Work out the finished part from the listing and answer in its coordinate system (mm). A direction names the side the tool comes from. Coordinates: 2 decimals unless noted, no trailing zeros. Order: outer loops, then holes, each group sorted by start corner. A loop starts at its lowest first (then second) coordinate and runs counter-clockwise, first axis right, second up.
```python
from build123d import *

# Parameters (mm, degrees)
SKETCH_1_W      = 5
SKETCH_1_H      = 5
SKETCH_1_W_2    = 3
SKETCH_1_H_2    = 3
EXTRUDE_1_DEPTH = 8
SKETCH_2_W      = 5
SKETCH_2_H      = 5
EXTRUDE_2_DEPTH = 2
SKETCH_3_W      = 10
SKETCH_3_H      = 2
EXTRUDE_3_DEPTH = 2
EXTRUDE_4_DEPTH = 2


with BuildPart() as part:
    # 草图1 → 凸台-拉伸1 (new body)
    with BuildSketch(Plane(origin=(0, 0, 0), x_dir=(0, 0, -1), z_dir=(1, 0, 0))):
        Rectangle(SKETCH_1_W, SKETCH_1_H)
        Rectangle(SKETCH_1_W_2, SKETCH_1_H_2, mode=Mode.SUBTRACT)
    extrude(amount=EXTRUDE_1_DEPTH)

    # 草图2 → 凸台-拉伸2 (add)
    with BuildSketch(Plane(origin=(8, 0, 0), x_dir=(0, 0, -1), z_dir=(1, 0, 0))):
        Rectangle(SKETCH_2_W, SKETCH_2_H)
    extrude(amount=EXTRUDE_2_DEPTH)

    # 草图3 → 凸台-拉伸3 (add)
    with BuildSketch(Plane.XZ.offset(2.5)):
        with Locations((5, 0)):
            Rectangle(SKETCH_3_W, SKETCH_3_H)
    extrude(amount=EXTRUDE_3_DEPTH)

    # 草图4 → 凸台-拉伸4 (add)
    with BuildSketch(Plane.XY.offset(1)):
        with BuildLine():
            Line((10, -4.5), (0, -4.5))
            Line((0, -4.5), (1.040402547, -12.634344629))
            ThreePointArc((1.040402547, -12.634344629), (8.203170669, -16.488433915), (9.535533906, -8.464466094))
            ThreePointArc((9.535533906, -8.464466094), (7.767766953, -8.464466094), (7.767766953, -10.232233047))
            ThreePointArc((7.767766953, -10.232233047), (5.996135796, -14.499997014), (4.237706296, -10.226776691))
            Line((4.237706296, -10.226776691), (7.30901916, -7.174394459))
            Line((7.30901916, -7.174394459), (10, -4.5))
        make_face()
    extrude(amount=-EXTRUDE_4_DEPTH)


solid = part.part
```
1. The part is cut by section C-C (y = 0.5). Determine the outline of the cut face in (x, z), plus the area to 3 significant figures.
2. For faces 4 (the flat face through (5, -8, -1)), 5 (the cylindrical face through (8.083, -16.545, 0.014)), 6 (the flat face through (5, 0, -2.5)), 7 (the flat face through (5, -2.5, 2)), 8 (the flat face through (4, 1.5, 0)), determine the directions among +Z, -Z, +X, -X, +Y, -Y from which every point of the face is accessible in a straight line to the end or side of a thin tool.
3. The part is cut by section A-A (x = 6). Determine the outline of the cut face in (y, z).
4. The part is cut by section D-D (z = 0.8). Determine the outline of the cut face in (x, y).
5. The part is cut by section B-B (y = -12). Determine the outline of the cut face in (x, z), plus the area to 3 significant figures.
6. Consider probe 1 along Z at (x, y) = (6, -0.75); probe 2 along Y at (x, z) = (6, 0.4); probe 3 along Y at (x, z) = (6.5, 0.3). Determine where each line is inside the solid, lowest interval first.
7. The mould has two halves that part along X. Classify faces 1 (the cylindrical face through (7.787, -8.445, 0.014)), 2 (the flat face through (5, 2.5, 0)), 3 (the flat face through (10, 0, 0)): released by +X, released by -X, zero draft, split by the parting line, or undercut.
8. Flat-ended cylindrical pins translate along their axes: pin 1 (5 mm diameter, centred on x = 7, y = -10, fed in from +Z); pin 2 (2 mm diameter, centred on y = -6, z = -0.5, fed in from -X); pin 3 (1.6 mm diameter, centred on x = 6.5, z = -2, fed in from -Y). Find the tip coordinate at first contact, or state that the pin passes through.
Worked out:
1. outline: (0, -2.5) - (10, -2.5) - (10, 2.5) - (0, 2.5) - (0, 1.5) - (8, 1.5) - (8, -1.5) - (0, -1.5) - close
1. area: 26.0 mm2
2. face 4: -Z, +X, -X, -Y
2. face 5: +Z, -Z
2. face 6: -Z, +X, -X, +Y, -Y
2. face 7: +Z, +X, -X, -Y
2. face 8: -X
3. outline: (-17, -1) - (-14.5, -1) - (-14.5, 1) - (-17, 1) - close; (-8.48, -1) - (-2.5, -1) - (-2.5, -2.5) - (2.5, -2.5) - (2.5, 2.5) - (-2.5, 2.5) - (-2.5, 1) - (-8.48, 1) - close; hole (-1.5, -1.5) - (1.5, -1.5) - (1.5, 1.5) - (-1.5, 1.5) - close
4. outline: (0, -4.5) - (1.04, -12.63) arc R5 ccw (long way) to (9.54, -8.46) arc R1.25 ccw to (7.77, -10.23) arc R2.5 cw (long way) to (4.24, -10.23) - (10, -4.5) - (10, 2.5) - (0, 2.5) - (0, 1.5) - (8, 1.5) - (8, -1.5) - (0, -1.5) - close
5. outline: (0.96, -1) - (3.5, -1) - (3.5, 1) - (0.96, 1) - close; (8.5, -1) - (11, -1) - (11, 1) - (8.5, 1) - close
5. area: 10.1 mm2
6. probe 1: z = -2.5 to -1.5, 1.5 to 2.5
6. probe 2: y = -17 to -14.5, -8.48 to -1.5, 1.5 to 2.5
6. probe 3: y = -16.97 to -14.45, -7.98 to -1.5, 1.5 to 2.5
7. face 1: undercut
7. face 2: zero draft
7. face 3: released by +X
8. pin 1: stops at z = 1
8. pin 2: stops at x = 0.06
8. pin 3: stops at y = -2.5
